Verification items for the finished model (mm, model axes). A direction names the side the tool comes from. Give positions to 0.01 mm unless a question says otherwise; leave off trailing zeros. Write each loop counter-clockwise with the first axis right and the second up, starting at its lowest first coordinate (ties: lowest second). Pieces come first, ordered by that corner, then holes. Notation, with made-up numbers: (78.25, 32) - (133.25, 32) arc R18 cw to (133.25, 38) - close; hole circle Ø11 at (49.25, -11). An arc over 180 degrees is marked (long way). Answer as a JSON object with one key per item and string values. Group by question number.
Item 1: Sectioned sample at D-D, the plane z = 10.5. Record the boundary of the cut face in (x, y).
Item 2: Sectioned sample at A-A, the plane x = 9. Record the boundary of the cut face in (y, z).
Item 3: Scan lines: line 1 along Y through (x, z) = (-9, 3.25); line 2 along Y through (x, z) = (9, 2.55); line 3 along X through (y, z) = (12.25, 3.2). Record each from-to range of solid material in increasing order. Write a range as [from, to].
Item 4: Tool access check on faces 5 (the face through (0, 0, 0)), 6 (the face through (9, 9, 9)), 7 (the face through (2.645, 11.198, 4.121)), 8 (the face through (0, 0, 14)). Record the directions out of +Z, -Z, +X, -X, +Y, -Y that give a thin tool (end or side, any length) a straight path to the whole face; none if there is none.
Item 5: Draft check along Y on faces 1 (the face through (8.675, -10.464, 7.028)), 2 (the face through (15, 0, 7)), 3 (the face through (-9, 9, 9)), 4 (the face through (0, 15, 7)). Enter one of: +Y half, -Y half, draft (parallel to the pull), parting line (faces both ways), or undercut.
Item 6: Go/stop test with flat-tipped pins: pin 1 (7 mm diameter, centred on x = -9, y = 9, fed in from +Z); pin 2 (1.8 mm diameter, centred on x = 9, y = -9, fed in from -Z); pin 3 (3 mm diameter, centred on x = -3.5, y = -4.5, fed in from -Z); pin 4 (2.5 mm diameter, centred on x = 9.5, y = 9.5, fed in from -Z). Record where each tip stops, or that it passes through.
Item 7: Sectioned sample at C-C, the plane z = 8.5. Record the boundary of the cut face in (x, y), and give its area (3 significant figures).
Item 8: Sectioned sample at B-B, the plane y = 2. Record the boundary of the cut face in (x, z).
```python
from build123d import *

# Parameters (mm, degrees)
SKETCH_1_W                = 30
SKETCH_1_H                = 30
EXTRUDE_1_DEPTH           = 14
SKETCH_2_R                = 8
SKETCH_2_R_2              = 7.5
EXTRUDE_2_DEPTH           = 2
SKETCH_3_R                = 2.5
CUT_EXTRUDE_1_DEPTH       = 15
HOLE_WIZARD_M3_1_D        = 2.5
HOLE_WIZARD_M3_1_DEPTH    = 7.5
HOLE_WIZARD_M3_1_TIP      = 0.751075774
HOLE_WIZARD_1_D           = 3
HOLE_WIZARD_1_DEPTH       = 9
HOLE_WIZARD_1_CBORE_D     = 6
HOLE_WIZARD_1_CBORE_DEPTH = 5


with BuildPart() as part:
    # 草图1 → 凸台-拉伸1 (new body)
    with BuildSketch(Plane.XY):
        Rectangle(SKETCH_1_W, SKETCH_1_H)
    extrude(amount=EXTRUDE_1_DEPTH)

    # 草图2 → 凸台-拉伸2 (add)
    with BuildSketch(Plane.XY.offset(14)):
        Circle(SKETCH_2_R)
        Circle(SKETCH_2_R_2, mode=Mode.SUBTRACT)
    extrude(amount=EXTRUDE_2_DEPTH)

    # 草图3 → 切除-拉伸1 (cut)
    with BuildSketch(Plane(origin=(0, 15, 0), x_dir=(1, 0, 0), z_dir=(0, 1, 0))):
        with Locations(Location((-3, -8.5, 0), (0, 0, 270))):
            Circle(SKETCH_3_R)
    extrude(amount=-CUT_EXTRUDE_1_DEPTH, mode=Mode.SUBTRACT)

    # M3 螺纹孔1
    with Locations(Plane(origin=(1.8, 15, 3.2), x_dir=(0, 0, 1), z_dir=(0, 1, 0))):
        with Locations((0, 0)):
            Hole(HOLE_WIZARD_M3_1_D / 2, depth=HOLE_WIZARD_M3_1_DEPTH)
            with Locations((0, 0, -(HOLE_WIZARD_M3_1_DEPTH + HOLE_WIZARD_M3_1_TIP / 2))):  # 118° drill point
                Cone(0, HOLE_WIZARD_M3_1_D / 2, HOLE_WIZARD_M3_1_TIP, mode=Mode.SUBTRACT)

    # 孔1
    with Locations(Plane(origin=(9, 8.916915074, 0), x_dir=(-1, 0, 0), z_dir=(0, 0, -1))):
        with Locations((0, 0), (18, 0.083084926), (18, -17.916915074), (0, -17.916915074)):
            CounterBoreHole(HOLE_WIZARD_1_D / 2, HOLE_WIZARD_1_CBORE_D / 2, HOLE_WIZARD_1_CBORE_DEPTH, depth=HOLE_WIZARD_1_DEPTH)


solid = part.part
```
Geometry check:
{
 "1": {"outline": "(-15, -15) - (15, -15) - (15, 15) - (-1.5, 15) - (-1.5, 0) - (-4.5, 0) - (-4.5, 15) - (-15, 15) - close"},
 "2": {"outline": "(-15, 0) - (-12, 0) - (-12, 5) - (-10.5, 5) - (-10.5, 9) - (-7.5, 9) - (-7.5, 5) - (-6, 5) - (-6, 0) - (5.92, 0) - (5.92, 5) - (7.42, 5) - (7.42, 9) - (10.42, 9) - (10.42, 5) - (11.92, 5) - (11.92, 0) - (15, 0) - (15, 14) - (-15, 14) - close"},
 "3": {"line 1": "[-15, -12], [-6, 6], [12, 15]", "line 2": "[-15, -12], [-6, 5.92], [11.92, 15]", "line 3": "[-15, 0.55], [3.05, 15]"},
 "4": {"face 5": "-Z, +X, -X, +Y, -Y", "face 6": "-Z", "face 7": "+Y", "face 8": "+Z"},
 "5": {"face 1": "undercut", "face 2": "draft", "face 3": "undercut", "face 4": "+Y half"},
 "6": {"pin 1": "z = 14", "pin 2": "z = 9", "pin 3": "z = 0", "pin 4": "z = 5"},
 "7": {"outline": "(-15, -15) - (15, -15) - (15, 15) - (-0.5, 15) - (-0.5, 0) - (-5.5, 0) - (-5.5, 15) - (-15, 15) - close; hole circle Ø3 at (-9, -9); hole circle Ø3 at (-9, 9); hole circle Ø3 at (9, -9); hole circle Ø3 at (9, 8.92)", "area": "797 mm^2"},
 "8": {"outline": "(-15, 0) - (15, 0) - (15, 14) - (7.75, 14) - (7.75, 16) - (7.23, 16) - (7.23, 14) - (-7.23, 14) - (-7.23, 16) - (-7.75, 16) - (-7.75, 14) - (-15, 14) - close; hole circle Ø5 at (-3, 8.5)"}
}
